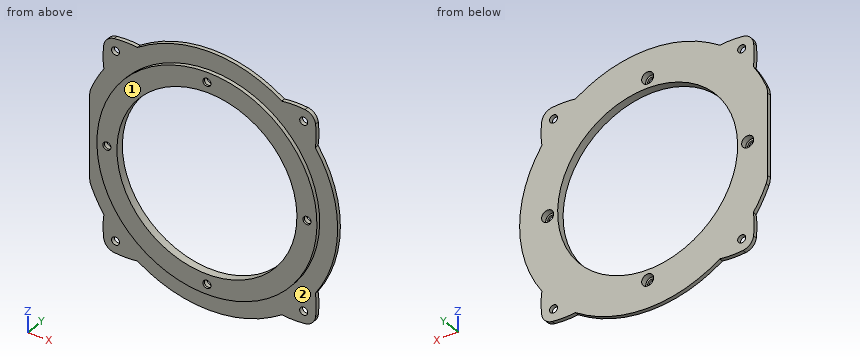
from build123d import *

# Parameters (mm, degrees)
SKETCH_1_R               = 55
SKETCH_1_R_2             = 45
EXTRUDE_1_DEPTH          = 4
EXTRUDE_START            = -4
SKETCH_2_R               = 64
SKETCH_2_R_2             = 55
EXTRUDE_2_DEPTH          = 2
SKETCH_3_R               = 3
CUT_EXTRUDE_1_DEPTH      = 3
PATTERN_CIRCULAR_1_COUNT = 4
SKETCH_4_R               = 2
CUT_EXTRUDE_2_DEPTH      = 91.559372789
PATTERN_CIRCULAR_2_COUNT = 4
SKETCH_5_R               = 2
EXTRUDE_3_DEPTH          = 2
CUT_EXTRUDE_3_DEPTH      = 91.598013365
CUT_EXTRUDE_3_DEPTH_BACK = 91.598013365
FILLET_1_R               = 10


with BuildPart() as part:
    # 草图1 → 凸台-拉伸1 (new body)
    with BuildSketch(Plane(origin=(0, 0, 0), x_dir=(1, 0, 0), z_dir=(0, 1, 0))):
        with Locations(Location((0, 0, 0), (0, 0, 270))):
            Circle(SKETCH_1_R)
        with Locations(Location((0, 0, 0), (0, 0, 270))):
            Circle(SKETCH_1_R_2, mode=Mode.SUBTRACT)
    extrude(amount=-EXTRUDE_1_DEPTH)

    # 草图2 → 凸台-拉伸2 (add)
    with BuildSketch(Plane(origin=(0, -4, 0), x_dir=(-1, 0, 0), z_dir=(0, -1, 0)).offset(EXTRUDE_START)):
        with Locations(Location((0, 0, 0), (0, 0, 90))):
            Circle(SKETCH_2_R)
        with Locations(Location((0, 0, 0), (0, 0, 270))):
            Circle(SKETCH_2_R_2, mode=Mode.SUBTRACT)
    extrude(amount=EXTRUDE_2_DEPTH)

    # 草图3 → 切除-拉伸1 (cut)
    with BuildSketch(Plane(origin=(0, 0, 0), x_dir=(1, 0, 0), z_dir=(0, 1, 0))):
        with Locations(Location((0, 50, 0), (0, 0, 270))):
            Circle(SKETCH_3_R)
    cut_extrude_1 = extrude(amount=-CUT_EXTRUDE_1_DEPTH, mode=Mode.SUBTRACT)

    # 阵列(圆周)1: 切除-拉伸1 ×4 about axis
    pattern_circular_1_axis = Axis((0, 0, 0), (0, 1, 0))
    for i in range(1, PATTERN_CIRCULAR_1_COUNT):
        add(cut_extrude_1.rotate(pattern_circular_1_axis, i * 360 / PATTERN_CIRCULAR_1_COUNT), mode=Mode.SUBTRACT)

    # 草图4 → 切除-拉伸2 (cut, through all)
    with BuildSketch(Plane(origin=(0, -3, 0), x_dir=(1, 0, 0), z_dir=(0, 1, 0))):
        with Locations(Location((0, 50, 0), (0, 0, 270))):
            Circle(SKETCH_4_R)
    cut_extrude_2 = extrude(amount=-CUT_EXTRUDE_2_DEPTH, mode=Mode.SUBTRACT)

    # 阵列(圆周)2: 切除-拉伸2 ×4 about axis
    pattern_circular_2_axis = Axis((0, 0, 0), (0, 1, 0))
    for i in range(1, PATTERN_CIRCULAR_2_COUNT):
        add(cut_extrude_2.rotate(pattern_circular_2_axis, i * 360 / PATTERN_CIRCULAR_2_COUNT), mode=Mode.SUBTRACT)

    # 草图5 → 凸台-拉伸3 (add)
    # profile 1 of 4: a face of its own
    with BuildSketch(Plane(origin=(0, 0, 0), x_dir=(1, 0, 0), z_dir=(0, 1, 0))):
        with BuildLine():
            ThreePointArc((47.70579193, 52.971441059), (51.25436151, 51.25436151), (52.971441059, 47.70579193))
            add(Edge.make_bspline(
                [(52.875879568, 36.057473011), (53.400264575, 39.842208211), (53.419874183, 43.855270087), (52.971441059, 47.70579193)],
                knots=[0, 0, 0, 0, 0.718259979, 0.718259979, 0.718259979, 0.718259979], degree=3))
            ThreePointArc((52.875879568, 36.057473011), (45.254833996, 45.254833996), (36.057473011, 52.875879568))
            add(Edge.make_bspline(
                [(36.057473011, 52.875879568), (39.842208211, 53.400264575), (43.855270087, 53.419874183), (47.70579193, 52.971441059)],
                knots=[0, 0, 0, 0, 0.718259979, 0.718259979, 0.718259979, 0.718259979], degree=3))
        make_face()
        with Locations(Location((47.022600949, 47.022600949, 0), (0, 0, 270))):
            Circle(SKETCH_5_R, mode=Mode.SUBTRACT)
    # profile 2 of 4: a face of its own
    with BuildSketch(Plane(origin=(0, 0, 0), x_dir=(1, 0, 0), z_dir=(0, 1, 0))):
        with BuildLine():
            ThreePointArc((52.971441059, -47.70579193), (51.25436151, -51.25436151), (47.70579193, -52.971441059))
            add(Edge.make_bspline(
                [(36.057473011, -52.875879568), (39.842208211, -53.400264575), (43.855270087, -53.419874183), (47.70579193, -52.971441059)],
                knots=[0, 0, 0, 0, 0.718259979, 0.718259979, 0.718259979, 0.718259979], degree=3))
            ThreePointArc((36.057473011, -52.875879568), (45.254833996, -45.254833996), (52.875879568, -36.057473011))
            add(Edge.make_bspline(
                [(52.875879568, -36.057473011), (53.400264575, -39.842208211), (53.419874183, -43.855270087), (52.971441059, -47.70579193)],
                knots=[0, 0, 0, 0, 0.718259979, 0.718259979, 0.718259979, 0.718259979], degree=3))
        make_face()
        with Locations(Location((47.022600949, -47.022600949, 0), (0, 0, 270))):
            Circle(SKETCH_5_R, mode=Mode.SUBTRACT)
    # profile 3 of 4: a face of its own
    with BuildSketch(Plane(origin=(0, 0, 0), x_dir=(1, 0, 0), z_dir=(0, 1, 0))):
        with BuildLine():
            ThreePointArc((-47.70579193, -52.971441059), (-51.25436151, -51.25436151), (-52.971441059, -47.70579193))
            add(Edge.make_bspline(
                [(-52.875879568, -36.057473011), (-53.400264576, -39.842208211), (-53.419874183, -43.855270087), (-52.971441059, -47.70579193)],
                knots=[0, 0, 0, 0, 0.718259979, 0.718259979, 0.718259979, 0.718259979], degree=3))
            ThreePointArc((-52.875879568, -36.057473011), (-45.254833996, -45.254833996), (-36.057473011, -52.875879568))
            add(Edge.make_bspline(
                [(-36.057473011, -52.875879568), (-39.842208211, -53.400264575), (-43.855270087, -53.419874183), (-47.70579193, -52.971441059)],
                knots=[0, 0, 0, 0, 0.718259979, 0.718259979, 0.718259979, 0.718259979], degree=3))
        make_face()
        with Locations(Location((-47.022600949, -47.022600949, 0), (0, 0, 270))):
            Circle(SKETCH_5_R, mode=Mode.SUBTRACT)
    # profile 4 of 4: a face of its own
    with BuildSketch(Plane(origin=(0, 0, 0), x_dir=(1, 0, 0), z_dir=(0, 1, 0))):
        with BuildLine():
            ThreePointArc((-52.971441059, 47.70579193), (-51.25436151, 51.25436151), (-47.70579193, 52.971441059))
            add(Edge.make_bspline(
                [(-36.057473011, 52.875879568), (-39.842208211, 53.400264576), (-43.855270087, 53.419874183), (-47.70579193, 52.971441059)],
                knots=[0, 0, 0, 0, 0.718259979, 0.718259979, 0.718259979, 0.718259979], degree=3))
            ThreePointArc((-36.057473011, 52.875879568), (-45.254833996, 45.254833996), (-52.875879568, 36.057473011))
            add(Edge.make_bspline(
                [(-52.875879568, 36.057473011), (-53.400264575, 39.842208211), (-53.419874183, 43.855270087), (-52.971441059, 47.70579193)],
                knots=[0, 0, 0, 0, 0.718259979, 0.718259979, 0.718259979, 0.718259979], degree=3))
        make_face()
        with Locations(Location((-47.022600949, 47.022600949, 0), (0, 0, 270))):
            Circle(SKETCH_5_R, mode=Mode.SUBTRACT)
    extrude(amount=-EXTRUDE_3_DEPTH)

    # 草图6 → 切除-拉伸3 (cut, two sides: drawn at the far end of the back side and taken through both)
    with BuildSketch(Plane(origin=(0, 0, 0), x_dir=(1, 0, 0), z_dir=(0, 1, 0)).offset(-CUT_EXTRUDE_3_DEPTH_BACK)):
        Polygon((-60, 26.714394046), (-60, -26.64509416), (-76.414310547, -26.64509416), (-74.893876556, 32.809859769), align=None)
    extrude(amount=CUT_EXTRUDE_3_DEPTH + CUT_EXTRUDE_3_DEPTH_BACK, mode=Mode.SUBTRACT)

    # 圆角1
    fillet_1_edges = [part.edges().sort_by_distance(p)[0] for p in [
        (-60, -1, 22.271057451),
        (-60, -1, -22.271057451),
    ]]
    fillet(fillet_1_edges, radius=FILLET_1_R)


solid = part.part
The model under review builds one solid part; all positions refer to its coordinate system, in mm. Face numbers are marked on the shaded views. A direction names the side the tool comes from. Coordinates: 2 decimals unless noted, no trailing zeros. Write each loop counter-clockwise with the first axis right and the second up, starting at its lowest first coordinate (ties: lowest second). Pieces come first, ordered by that corner, then holes. Notation, with made-up numbers: (-2, 89) - (55, 89) arc R19 ccw to (55, 101) - close; hole circle Ø6 at (-20.75, 22.25). An arc over 180 degrees is marked (long way). Answer as CSV lines item,"result".
(1) We need section C-C (z = 26). Give the boundary of the cut face in (x, y).
Data:
outline,"(-58.48, -2) - (-48.47, -2) - (-48.47, -4) - (-36.73, -4) - (-36.73, 0) - (-58.48, 0) - close; (36.73, -4) - (48.47, -4) - (48.47, -2) - (58.48, -2) - (58.48, 0) - (36.73, 0) - close"
(2) Tool access review of the marked faces 1 and 2: name each direction out of +Z, -Z, +X, -X, +Y, -Y from which nothing blocks a thin tool from reaching the whole face with its end or side.
Data:
face 1,"+Z, -Z, +X, -X, -Y"
face 2,"-Y"
(3) We need section D-D (x = 28). Give the boundary of the cut face in (y, z).
Data:
outline,"(-4, -47.34) - (-2, -47.34) - (-2, -57.55) - (0, -57.55) - (0, -35.23) - (-4, -35.23) - close; (-4, 35.23) - (0, 35.23) - (0, 57.55) - (-2, 57.55) - (-2, 47.34) - (-4, 47.34) - close"
(4) We need section B-B (x = 0). Give the boundary of the cut face in (y, z), plus the area to 3 significant figures.
Data:
outline,"(-4, -55) - (-2, -55) - (-2, -64) - (0, -64) - (0, -53) - (-3, -53) - (-3, -52) - (-4, -52) - close; (-4, -48) - (-3, -48) - (-3, -47) - (0, -47) - (0, -45) - (-4, -45) - close; (-4, 45) - (0, 45) - (0, 47) - (-3, 47) - (-3, 48) - (-4, 48) - close; (-4, 52) - (-3, 52) - (-3, 53) - (0, 53) - (0, 64) - (-2, 64) - (-2, 55) - (-4, 55) - close"
area,"72.0 mm2"
(5) For line 1 along Z through (x, y) = (46.5, -0.2); line 2 along Z through (x, y) = (47.5, -0.45); line 3 along Z through (x, y) = (2.5, -0.2), list the stretches that pass through material, from the lowest coordinate up. Write a range as [from, to].
Data:
line 1,"z = [-53.1, -48.95], [-45.09, 45.09], [48.95, 53.1]"
line 2,"z = [-52.99, -48.96], [-45.08, -1.66], [1.66, 45.08], [48.96, 52.99]"
line 3,"z = [-63.95, -51.66], [-48.34, -44.93], [44.93, 48.34], [51.66, 63.95]"
(6) Clearance check with flat-ended pins moving along their axes: pin 1 Ø1.8 at (x, z) = (1.5, 49.5) entering from +Y; pin 2 Ø4.5 at (x, z) = (-50, 0) entering from -Y; pin 3 Ø1.5 at (y, z) = (-1, 50.5) entering from -X. State where each tip first meets the part, or that it passes through.
Data:
pin 1,"stops at y = -3"
pin 2,"stops at y = -4"
pin 3,"stops at x = -52.35"
(7) We need section A-A (z = 0). Give the boundary of the cut face in (x, y).
Data:
outline,"(-60, -2) - (-55, -2) - (-55, -4) - (-52, -4) - (-52, -3) - (-53, -3) - (-53, 0) - (-60, 0) - close; (-48, -4) - (-45, -4) - (-45, 0) - (-47, 0) - (-47, -3) - (-48, -3) - close; (45, -4) - (48, -4) - (48, -3) - (47, -3) - (47, 0) - (45, 0) - close; (52, -4) - (55, -4) - (55, -2) - (64, -2) - (64, 0) - (53, 0) - (53, -3) - (52, -3) - close"
